Here's how the part is built. I have some questions about the finished solid (model axes, mm). A direction names the side the tool comes from. Round coordinates to 2 decimals unless told otherwise and drop trailing zeros. Order: outer loops, then holes, each group sorted by start corner. A loop starts at its lowest first (then second) coordinate and runs counter-clockwise, first axis right, second up. Notation, with made-up numbers: (70, 70) - (108, 70) arc R30 ccw to (108, 96) - close; hole circle Ø4 at (72, -37.5). An arc over 180 degrees is marked (long way). One line per item, written item: value.
from build123d import *

# Parameters (mm, degrees)
ESQUISSE1_W             = 20
ESQUISSE1_H             = 9.6
BOSS_EXTRU_1_DEPTH      = 6.4
ESQUISSE2_R             = 1.175
ENL_V_MAT_EXTRU_1_DEPTH = 6.4
BOSS_EXTRU_66_DEPTH     = 6.4
ESQUISSE5_W             = 0.63
ESQUISSE5_H             = 3.33
BOSS_EXTRU_67_DEPTH     = 4.01
ESQUISSE6_R             = 0.6
ENL_V_MAT_EXTRU_2_DEPTH = 19.01


with BuildPart() as part:
    # Esquisse1 → Boss.-Extru.1 (new body)
    with BuildSketch(Plane.XY):
        with Locations((11.361848554, 25.841592458)):
            Rectangle(ESQUISSE1_W, ESQUISSE1_H)
    extrude(amount=BOSS_EXTRU_1_DEPTH)

    # Esquisse2 → Enlèv. mat.-Extru.1 (cut)
    with BuildSketch(Plane.XY.offset(6.4)):
        with Locations((16.186848554, 24.016592458)):
            Circle(ESQUISSE2_R)
        with Locations((6.536848554, 24.016592458)):
            Circle(ESQUISSE2_R)
    extrude(amount=-ENL_V_MAT_EXTRU_1_DEPTH, mode=Mode.SUBTRACT)

    # Esquisse4 → Boss.-Extru.66 (add)
    with BuildSketch(Plane.XY.offset(6.4)):
        Polygon((1.361848554, 32.424730159), (1.361848554, 30.641592458), (9.361848554, 30.641592458), (9.24123613, 31.809658088), (7.392325504, 31.809658088), (7.392325504, 33.099658088), (5.512325504, 33.099658088), (5.512325504, 31.809658088), (2.052325504, 31.809658088), (2.052325504, 32.309658088), (21.361848554, 37.201602535), (21.361848554, 37.491602535), align=None)
    extrude(amount=-BOSS_EXTRU_66_DEPTH)

    # Esquisse5 → Boss.-Extru.67 (add)
    with BuildSketch(Plane.XZ.offset(-21.041592458)):
        with Locations((3.256848554, 3.185)):
            Rectangle(ESQUISSE5_W, ESQUISSE5_H)
        with Locations((11.386848554, 3.185)):
            Rectangle(ESQUISSE5_W, ESQUISSE5_H)
        with Locations((19.466848554, 3.185)):
            Rectangle(ESQUISSE5_W, ESQUISSE5_H)
    extrude(amount=BOSS_EXTRU_67_DEPTH)

    # Esquisse6 → Enlèv. mat.-Extru.2 (cut)
    with BuildSketch(Plane.ZY.offset(-2.941848554)):
        with Locations((3.2, 18.531592458)):
            Circle(ESQUISSE6_R)
    extrude(amount=-ENL_V_MAT_EXTRU_2_DEPTH, mode=Mode.SUBTRACT)


solid = part.part
Q1. Which directions (+Z, -Z, +X, -X, +Y, -Y) give clear straight access to the entire face, cutting with the end or side of a thin tool? Please do faces 4 (the flat face through (19.152, 19, 4)), 5 (the flat face through (2.942, 19, 4)), 6 (the flat face through (6, 33.1, 3)), 7 (the flat face through (19.782, 19, 4)), 8 (the flat face through (11.57, 34.72, 3.24)).
Results list:
face 4: +Z, -Z, -Y
face 5: +Z, -Z, -X, -Y
face 6: +Z, -Z, +X
face 7: +Z, -Z, +X, -Y
face 8: +Z, -Z
Q2. If we section it at C-C, the plane z = 4.25: Please give me the cut outline in (x, y) (3 decimals).
Results list:
outline: (1.362, 21.042) - (2.942, 21.042) - (2.942, 17.032) - (3.572, 17.032) - (3.572, 21.042) - (11.072, 21.042) - (11.072, 17.032) - (11.702, 17.032) - (11.702, 21.042) - (19.152, 21.042) - (19.152, 17.032) - (19.782, 17.032) - (19.782, 21.042) - (21.362, 21.042) - (21.362, 30.642) - (9.362, 30.642) - (9.241, 31.81) - (7.392, 31.81) - (7.392, 33.1) - (5.512, 33.1) - (5.512, 31.81) - (2.052, 31.81) - (2.052, 32.31) - (21.362, 37.202) - (21.362, 37.492) - (1.362, 32.425) - close; hole circle Ø2.35 at (6.537, 24.017); hole circle Ø2.35 at (16.187, 24.017)
Q3. If we section it at B-B, the plane x = 8.75: Please give me the cut outline in (y, z), then the cut area to 3 significant figures.
Results list:
outline: (21.04, 0) - (31.81, 0) - (31.81, 6.4) - (21.04, 6.4) - close; (34.01, 0) - (34.3, 0) - (34.3, 6.4) - (34.01, 6.4) - close
area: 70.8 mm²
Q4. We'd pull the mould along X, two halves only. Please class faces 1 (the flat face through (3.572, 19, 4)), 2 (the flat face through (11.502, 34.994, 3.245)), 3 (the flat face through (11, 28, 6.4)): released by +X, released by -X, zero draft, split by the parting line, or undercut.
Results list:
face 1: undercut
face 2: released by -X
face 3: zero draft
Q5. If I drill on line 1 along Y through (x, z) = (7.5, 4.25); line 2 along Y through (x, z) = (15.75, 5); line 3 along Z through (x, y) = (11.5, 20), over which ranges is the centre line in solid material (lowest first)?
Results list:
line 1: 21.04 to 23.34, 24.69 to 31.81, 33.69 to 33.98
line 2: 21.04 to 22.93, 25.11 to 30.64, 35.78 to 36.07
line 3: 1.52 to 4.85
Q6. If we section it at D-D, the plane x = 6.25: Please give me the cut outline in (y, z).
Results list:
outline: (21.04, 0) - (22.88, 0) - (22.88, 6.4) - (21.04, 6.4) - close; (25.16, 0) - (33.1, 0) - (33.1, 6.4) - (25.16, 6.4) - close; (33.37, 0) - (33.66, 0) - (33.66, 6.4) - (33.37, 6.4) - close
Q7. If we section it at A-A, the plane y = 20.5: Please give me the cut outline in (x, z), then the cut area to 3 significant figures.
Results list:
outline: (2.94, 1.52) - (3.57, 1.52) - (3.57, 4.85) - (2.94, 4.85) - close; (11.07, 1.52) - (11.7, 1.52) - (11.7, 4.85) - (11.07, 4.85) - close; (19.15, 1.52) - (19.78, 1.52) - (19.78, 4.85) - (19.15, 4.85) - close
area: 6.29 mm²
Q8. Will these pins go through, and if not, where does the flat tip stop? pin 1 (1.5 mm diameter, centred on x = 7, z = 4, fed in from +Y); pin 2 (1.5 mm diameter, centred on y = 32.5, z = 3.5, fed in from +X); pin 3 (0.5 mm diameter, centred on x = 11.5, y = 18.5, fed in from +Z).
Results list:
pin 1: y = 34.04
pin 2: x = 9.25
pin 3: z = 4.85
